Work out the finished part from the listing and answer in its coordinate system (mm). A direction names the side the tool comes from. Round coordinates to 2 decimals unless told otherwise and drop trailing zeros. Write each loop counter-clockwise with the first axis right and the second up, starting at its lowest first coordinate (ties: lowest second). Pieces come first, ordered by that corner, then holes. Notation, with made-up numbers: (33, 43.5) - (40, 43.5) arc R16 ccw to (40, 73.5) - close; hole circle Ø8 at (79.25, 82.5). An arc over 180 degrees is marked (long way). Answer as a JSON object with one key per item and string values.
```python
from build123d import *

# Parameters (mm, degrees)
SKETCH_1_W          = 6
SKETCH_1_H          = 14
EXTRUDE_1_DEPTH     = 23
CHAMFER_1_SIZE      = 1
SKETCH_2_W          = 2.5
SKETCH_2_H          = 3.5
EXTRUDE_2_DEPTH     = 15
CHAMFER_2_SIZE      = 0.5
CHAMFER_3_SIZE      = 1
SKETCH_3_R          = 2.35
CUT_EXTRUDE_1_DEPTH = 5


with BuildPart() as part:
    # 스케치1 → 보스-돌출1 (new body)
    with BuildSketch(Plane.XY):
        Rectangle(SKETCH_1_W, SKETCH_1_H)
    extrude(amount=EXTRUDE_1_DEPTH)

    # 모따기1
    chamfer_1_edges = [part.edges().sort_by_distance(p)[0] for p in [
        (3, -7, 11.5),
        (-3, -7, 11.5),
        (-3, 7, 11.5),
        (3, 7, 11.5),
    ]]
    chamfer(chamfer_1_edges, length=CHAMFER_1_SIZE)

    # 스케치2 → 보스-돌출2 (add)
    with BuildSketch(Plane.XY):
        with Locations((4.25, 4.25)):
            Rectangle(SKETCH_2_W, SKETCH_2_H)
        with Locations((4.25, -4.25)):
            Rectangle(SKETCH_2_W, SKETCH_2_H)
        with Locations((-4.25, -4.25)):
            Rectangle(SKETCH_2_W, SKETCH_2_H)
        with Locations((-4.25, 4.25)):
            Rectangle(SKETCH_2_W, SKETCH_2_H)
    extrude(amount=EXTRUDE_2_DEPTH)

    # 모따기2
    chamfer_2_edges = [part.edges().sort_by_distance(p)[0] for p in [
        (-4.25, -6, 15),
        (-4.25, -2.5, 15),
        (-4.25, 2.5, 15),
        (-4.25, 6, 15),
        (-4.25, 2.5, 0),
        (-4.25, 6, 0),
        (-4.25, -6, 0),
        (-4.25, -2.5, 0),
        (4.25, -2.5, 0),
        (4.25, -2.5, 15),
        (4.25, -6, 0),
        (4.25, -6, 15),
        (4.25, 2.5, 0),
        (4.25, 2.5, 15),
        (4.25, 6, 0),
        (4.25, 6, 15),
    ]]
    chamfer(chamfer_2_edges, length=CHAMFER_2_SIZE)

    # 모따기3
    chamfer_3_edges = [part.edges().sort_by_distance(p)[0] for p in [
        (0, -7, 23),
        (-3, 0, 23),
        (3, 0, 23),
        (0, 7, 23),
        (-2.5, 6.5, 23),
        (2.5, 6.5, 23),
        (2.5, -6.5, 23),
        (-2.5, -6.5, 23),
    ]]
    chamfer(chamfer_3_edges, length=CHAMFER_3_SIZE)

    # 스케치3 → 컷-돌출1 (cut)
    with BuildSketch(Plane(origin=(0, 0, 0), x_dir=(-1, 0, 0), z_dir=(0, 0, -1))):
        with Locations((0, 3.5)):
            Circle(SKETCH_3_R)
    extrude(amount=-CUT_EXTRUDE_1_DEPTH, mode=Mode.SUBTRACT)


solid = part.part
```
Item 1: A cutting plane is placed at D-D (z = 13.5). Write down the section's boundary in (x, y), and give its area (3 significant figures).
Results found:
{"outline": "(-5.5, -6) - (-3, -6) - (-2, -7) - (2, -7) - (3, -6) - (5.5, -6) - (5.5, -2.5) - (3, -2.5) - (3, 2.5) - (5.5, 2.5) - (5.5, 6) - (3, 6) - (2, 7) - (-2, 7) - (-3, 6) - (-5.5, 6) - (-5.5, 2.5) - (-3, 2.5) - (-3, -2.5) - (-5.5, -2.5) - close", "area": "117 mm²"}
Item 2: A cutting plane is placed at B-B (y = 3.5). Write down the section's boundary in (x, z), and give its area (4 significant figures).
Results found:
{"outline": "(-5.5, 0) - (-2.35, 0) - (-2.35, 5) - (2.35, 5) - (2.35, 0) - (5.5, 0) - (5.5, 15) - (3, 15) - (3, 22) - (2, 23) - (-2, 23) - (-3, 22) - (-3, 15) - (-5.5, 15) - close", "area": "188.5 mm²"}
Item 3: Determine the mould class of faces 4 (the flat face through (-4, -6, 7)), 5 (the flat face through (-3, 0, 13)), 6 (the flat face through (-4, 6, 7)) for opening direction Y: pulls with the +Y half, pulls with the -Y half, needs draft (parallel to the pull), parting line crosses it, or undercut.
Results found:
{"face 4": "pulls with the -Y half", "face 5": "undercut", "face 6": "pulls with the +Y half"}
Item 4: Consider line 1 along Y through (x, z) = (0, 2); line 2 along X through (y, z) = (-0.25, 4); line 3 along Y through (x, z) = (4.75, 5.25). Determine where each line is inside the solid, lowest interval first.
Results found:
{"line 1": "-7 to 1.15, 5.85 to 7", "line 2": "-3 to 3", "line 3": "-6 to -2.5, 2.5 to 6"}
Item 5: A cutting plane is placed at A-A (x = -4.5). Write down the section's boundary in (y, z).
Results found:
{"outline": "(-6, 0.5) - (-5.5, 0) - (-3, 0) - (-2.5, 0.5) - (-2.5, 14.5) - (-3, 15) - (-5.5, 15) - (-6, 14.5) - close; (2.5, 0.5) - (3, 0) - (5.5, 0) - (6, 0.5) - (6, 14.5) - (5.5, 15) - (3, 15) - (2.5, 14.5) - close"}
Item 6: A cutting plane is placed at C-C (x = 0). Write down the section's boundary in (y, z), and give its area (4 significant figures).
Results found:
{"outline": "(-7, 0) - (1.15, 0) - (1.15, 5) - (5.85, 5) - (5.85, 0) - (7, 0) - (7, 22) - (6, 23) - (-6, 23) - (-7, 22) - close", "area": "297.5 mm²"}
Item 7: Each of these flat-tipped pins is pushed along its axis until it touches: P1, Ø0.8, axis at x = -4.5, z = 6.5, coming from the +Y side; P2, Ø0.8, axis at x = 4, y = 3.5, coming from the +Z side; P3, Ø4, axis at x = 0, y = 3.5, coming from the -Z side; P4, Ø6, axis at x = 4, z = 6.5, coming from the +Y side. Where does it stop, or does it pass through?
Results found:
{"P1": "y = 6", "P2": "z = 15", "P3": "z = 5", "P4": "y = 7"}
Item 8: For faces 1 (the flat face through (4, -2.5, 7)), 2 (the flat face through (-4, -4, 15)), 3 (the flat face through (-4, -2.5, 7)), determine the directions among +Z, -Z, +X, -X, +Y, -Y from which every point of the face is accessible in a straight line to the end or side of a thin tool.
Results found:
{"face 1": "+Z, -Z, +X", "face 2": "+Z, -X, +Y, -Y", "face 3": "+Z, -Z, -X"}
